from build123d import *

# Parameters (mm, degrees)
F1_DEPTH = 66.04
F2_R     = 33.02
F3_R     = 33.01999
F4_R     = 16.51
F5_DEPTH = 34.544
F7_DEPTH = 25.4


# Not quite as in the source:
# - a fillet or chamfer is up to 0.001 mm smaller than in the source, because OpenCascade refuses the exact size


with BuildPart() as f1:
    # F0 (on Front) → F1 (new body)
    with BuildSketch(Plane.XZ):
        Polygon((0, 86.36), (0, 0), (38.608, 0), (38.608, 19.304), (19.304, 19.304), (19.304, 86.36), align=None)
    extrude(amount=F1_DEPTH)

    # F2
    f2_edges = [f1.edges().sort_by_distance(p)[0] for p in [
        (9.652, 0, 86.36),
    ]]
    fillet(f2_edges, radius=F2_R)

    # F3 (radius 33.02 in the source; OpenCascade refuses exactly that, so slightly less here)
    f3_edges = [f1.edges().sort_by_distance(p)[0] for p in [
        (9.652, -66.04, 86.36),
    ]]
    fillet(f3_edges, radius=F3_R)

    # F4 (on face) → F5 (cut)
    with BuildSketch(Plane.YZ.offset(19.304)):
        with Locations((-33.02, 53.34)):
            Circle(F4_R)
    extrude(amount=-F5_DEPTH, mode=Mode.SUBTRACT)

    # F6 (on face) → F7 (cut)
    with BuildSketch(Plane.XY.offset(19.304)):
        Polygon((38.608, -47.244), (38.608, -33.02), (38.608, -18.796), (28.956, -18.796), (28.956, -47.244), align=None)
    extrude(amount=-F7_DEPTH, mode=Mode.SUBTRACT)


solid = f1.part
Work out the finished part from the listing and answer in its coordinate system (mm). A direction names the side the tool comes from. Give positions to 0.01 mm unless a question says otherwise; leave off trailing zeros. Loops run counter-clockwise (first coordinate to the right, second up) from the corner with the lowest first, then second, coordinate; pieces in that order, holes last. Notation, with made-up numbers: (62.25, 82.25) - (120.25, 82.25) arc R16 ccw to (120.25, 107.25) - close; hole circle Ø10 at (24, 66.5). An arc over 180 degrees is marked (long way). Answer in a Markdown table with one row per item. Add a question column.
Q1. The part is cut by section A-A (x = 35). Determine the outline of the cut face in (y, z).
Q2. Determine the mould class of faces 1 (the cylindrical face through (9.517, -56.111, 76.944)), 2 (the flat face through (15, 0, 21)), 3 (the flat face through (34, -47.244, 10)) for opening direction Y: released by +Y, released by -Y, zero draft, split by the parting line, or undercut.
Q3. A tool of negligible diameter and unlimited length cuts with its end or side. For faces 4 (the flat face through (19.304, -25, 37)), 5 (the flat face through (0, -33, 34)), 6 (the flat face through (28.956, -33, 10)), from which of +Z, -Z, +X, -X, +Y, -Y can it reach the whole face along a straight path? Write none if from no direction.
Q4. The part is cut by section C-C (z = 11). Determine the outline of the cut face in (x, y).
Q5. The part is cut by section B-B (z = 64). Determine the outline of the cut face in (x, y).
Q6. The part is cut by section D-D (y = -22.5). Determine the outline of the cut face in (x, z), and give its area (3 significant figures).
Q7. Consider line 1 along X through (y, z) = (-40.5, 8); line 2 along X through (y, z) = (-4, 22.5); line 3 along Y through (x, z) = (14, 52). Determine where each line is inside the solid, lowest interval first.
Q8. Each of these flat-tipped pins is pushed along its axis until it touches: P1, Ø4, axis at x = 34.5, y = -54, coming from the -Z side; P2, Ø15.5, axis at x = 30.5, y = -48, coming from the +Z side; P3, Ø8, axis at y = -32, z = 15, coming from the +X side; P4, Ø5, axis at x = 15.5, y = -45, coming from the +Z side. Where does it stop, or does it pass through?
Solution:
| question | item | result |
|---|---|---|
| 1 | outline | (-66.04, 0) - (-47.24, 0) - (-47.24, 19.3) - (-66.04, 19.3) - close; (-18.8, 0) - (0, 0) - (0, 19.3) - (-18.8, 19.3) - close |
| 2 | face 1 | released by -Y |
| 2 | face 2 | released by +Y |
| 2 | face 3 | undercut |
| 3 | face 4 | +Z, +X, +Y, -Y |
| 3 | face 5 | +Z, -Z, -X, +Y, -Y |
| 3 | face 6 | +Z, -Z, +X |
| 4 | outline | (0, -66.04) - (38.61, -66.04) - (38.61, -47.24) - (28.96, -47.24) - (28.96, -18.8) - (38.61, -18.8) - (38.61, 0) - (0, 0) - close |
| 5 | outline | (0, -64.27) - (19.3, -64.27) - (19.3, -45.63) - (0, -45.63) - close; (0, -20.41) - (19.3, -20.41) - (19.3, -1.77) - (0, -1.77) - close |
| 6 | outline | (0, 0) - (28.96, 0) - (28.96, 19.3) - (19.3, 19.3) - (19.3, 40.62) - (0, 40.62) - close; (0, 66.06) - (19.3, 66.06) - (19.3, 84.64) - (0, 84.64) - close |
| 6 | area | 1,330 mm² |
| 7 | line 1 | x = 0 to 28.96 |
| 7 | line 2 | x = 0 to 19.3 |
| 7 | line 3 | y = -66.04 to -49.48, -16.56 to 0 |
| 8 | P1 | stops at z = 0 |
| 8 | P2 | stops at z = 19.3 |
| 8 | P3 | stops at x = 28.96 |
| 8 | P4 | stops at z = 84.97 |
